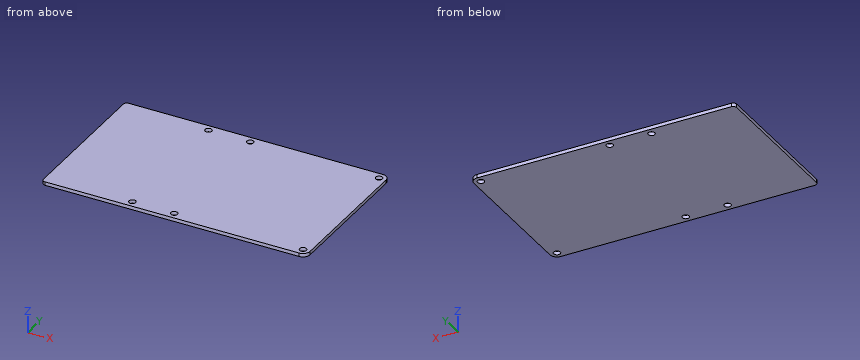
Autodesk Inventor part; units mm, degrees
ref_plane "YZ Plane" through (0, 0, 0) normal (1, 0, 0) x (0, 1, 0)
ref_plane "XZ Plane" through (0, 0, 0) normal (0, 1, 0) x (-1, 0, 0)
ref_plane "XY Plane" through (0, 0, 0) normal (0, 0, 1) x (1, 0, 0)
sketch "Sketch1" plane through (0, 0, 0) normal (0, 0, 1) x (1, 0, 0)
  line L0 (0, 97.79) -> (0, -97.79)
  line L1 (-200.025, 0) -> (200.025, 0)
  line L2 (142.875, -69.85) -> (-142.875, -69.85)
  line L3 (-142.875, -69.85) -> (-142.875, 69.85)
  line L4 (-142.875, 69.85) -> (142.875, 69.85)
  line L5 (142.875, 69.85) -> (142.875, -69.85)
  line L6 (142.875, -69.85) -> (-142.875, 69.85) construction
  line L7 (-142.875, -69.85) -> (142.875, 69.85) construction
  line L8 (-136.525, -63.5) -> (136.525, -63.5) construction
  line L9 (136.525, -63.5) -> (136.525, 63.5) construction
  line L10 (136.525, 63.5) -> (-136.525, 63.5) construction
  line L11 (-136.525, 63.5) -> (-136.525, -63.5) construction
  line L12 (-136.525, -63.5) -> (136.525, 63.5) construction
  line L13 (136.525, -63.5) -> (-136.525, 63.5) construction
  line L14 (-100.965, -14.2875) -> (-114.935, -14.2875)
  line L15 (-114.935, -14.2875) -> (-114.935, 14.2875)
  line L16 (-114.935, 14.2875) -> (-100.965, 14.2875)
  line L17 (-100.965, 14.2875) -> (-100.965, -14.2875)
  line L18 (-100.965, -14.2875) -> (-114.935, 14.2875) construction
  line L19 (-114.935, -14.2875) -> (-100.965, 14.2875) construction
  circle A0 centre (44.45, 31.75) radius 10.795
  circle A1 centre (44.45, -31.75) radius 10.795
  circle A2 centre (95.25, 0) radius 11.303
  circle A3 centre (95.25, 0) radius 30 construction
  line L20 (-64.135, -14.2875) -> (-50.165, -14.2875)
  line L21 (-50.165, -14.2875) -> (-50.165, 14.2875)
  line L22 (-50.165, 14.2875) -> (-64.135, 14.2875)
  line L23 (-64.135, 14.2875) -> (-64.135, -14.2875)
  line L24 (-64.135, -14.2875) -> (-50.165, 14.2875) construction
  line L25 (-50.165, -14.2875) -> (-64.135, 14.2875) construction
  line L26 (7.9375, -6.985) -> (-20.6375, -6.985)
  line L27 (-20.6375, -6.985) -> (-20.6375, 6.985)
  line L28 (-20.6375, 6.985) -> (7.9375, 6.985)
  line L29 (7.9375, 6.985) -> (7.9375, -6.985)
  line L30 (7.9375, -6.985) -> (-20.6375, 6.985) construction
  line L31 (-20.6375, -6.985) -> (7.9375, 6.985) construction
  point P0 (0, 0)
  point P1 (-107.95, 0)
  point P2 (95.25, 14.732)
  point P3 (95.25, -14.732)
  point P4 (-19.05, 63.5)
  point P5 (-19.05, -63.5)
  point P6 (19.05, -63.5)
  point P7 (19.05, 63.5)
  point P8 (-57.15, 0)
  point P9 (-6.35, 0)
  dimension "d0" = 285.75
  dimension "d1" = 139.7
  dimension "d4" = 6.35
  dimension "d5" = 6.35
  dimension "d6" = 13.97
  dimension "d7" = 28.575
  dimension "d15" = 0
  dimension "d16" = 21.59
  dimension "d20" = 22.606
  dimension "d22" = 60
  dimension "d33" = 47.625
  dimension "d34" = 14.732
  dimension "d35" = 14.732
  dimension "d43" = 34.925
  dimension "d44" = 31.75
  dimension "d45" = 31.75
  dimension "d46" = 152.4
  dimension "d47" = 50.8
  dimension "d48" = 19.05
  dimension "d49" = 19.05
  dimension "d50" = 50.8
  dimension "d51" = 50.8
extrude "Extrusion1" add sketch "Sketch1" along normal blind 3.175 contours L4 L5 L1 A2 L29 L28 L0 | L0 L28 L27 L1 L21 L22 L23 L17 L16 L15 L3 L4 | L28 L29 L1 L0 | L0 L1 L27 L28 | L1 L29 L26 L0 | L0 L26 L27 L1 | L1 L15 L14 L17 L23 L20 L21 L27 L26 L0 L2 L3 | L5 L2 L0 L26 L29 L1 A2 | L15 L16 L17 L1 | L1 L17 L14 L15 | A2 L1 | L1 A2 | L21 L20 L23 L1 | L1 L23 L22 L21 | A0 | A1
hole "Hole1" at (-136.525, 63.5, 0) at (-136.525, -63.5, 0) at (136.525, 63.5, 0) at (136.525, -63.5, 0) at (19.05, -63.5, 0) at (-19.05, 63.5, 0) at (19.05, 63.5, 0) at (-19.05, -63.5, 0) direction (0, 0, 1) diameter 6.096 end through all
fillet "Fillet1" radius 6.35 4 edges at (142.875, -69.85, 1.5875) (142.875, 69.85, 1.5875) (-142.875, -69.85, 1.5875) (-142.875, 69.85, 1.5875)
hole "Hole2" [suppressed]
sketch "Sketch2" plane through (0, 0, 3.175) normal (0, 0, 1) x (1, 0, 0)
  line L0 (0, 97.79) -> (0, -97.79)
  line L1 (-200.025, 0) -> (200.025, 0)
  line L2 (-98.425, -76.2) -> (-142.875, -76.2)
  line L3 (-142.875, -76.2) -> (-142.875, 76.2)
  line L4 (-142.875, 76.2) -> (-98.425, 76.2)
  line L5 (-98.425, 76.2) -> (-98.425, -76.2)
  line L6 (-98.425, -76.2) -> (-142.875, 76.2) construction
  line L7 (-142.875, -76.2) -> (-98.425, 76.2) construction
  line L8 (-142.875, 63.5) -> (-142.875, -63.5)
  point P0 (0, 0)
  point P1 (-120.65, 0)
  dimension "d52" = 0
  dimension "d53" = 44.45
  dimension "d54" = 152.4
extrude "Extrusion2" cut sketch "Sketch2" against normal blind 25.4
fillet "Fillet2" radius 3.175 2 edges at (-98.425, 69.85, 1.5875) (-98.425, -69.85, 1.5875)
Input: part model. Units: mm. Frame: model coordinates. Coordinates: 2 decimals unless noted, no trailing zeros. Write each loop counter-clockwise with the first axis right and the second up, starting at its lowest first coordinate (ties: lowest second). Pieces come first, ordered by that corner, then holes.
1) Material intervals for line 1 along X through (y, z) = (-63.5, 1.15) (3 decimals); line 2 along Y through (x, z) = (-19.05, 1.15), sorted ascending.
2) Section A-A on x = 19.05. Output: boundary loops of the cut face in (y, z) (3 decimals), and give its area (3 significant figures).
3) Pin query (flat end, axial travel): pin 1 Ø8 at (x, y) = (-19.05, -63.5) entering from -Z. Return the tip coordinate at first contact, or that it passes through.
Check result:
1. line 1: x = -98.425 to -22.098, -16.002 to 16.002, 22.098 to 133.477, 139.573 to 142.875
1. line 2: y = -69.85 to -66.55, -60.45 to 60.45, 66.55 to 69.85
2. outline: (-69.85, 0) - (-66.548, 0) - (-66.548, 3.175) - (-69.85, 3.175) - close; (-60.452, 0) - (60.452, 0) - (60.452, 3.175) - (-60.452, 3.175) - close; (66.548, 0) - (69.85, 0) - (69.85, 3.175) - (66.548, 3.175) - close
2. area: 405 mm2
3. pin 1: stops at z = 0
